Part model, mm, in its own coordinate system. A direction names the side the tool comes from. Round coordinates to 2 decimals unless told otherwise and drop trailing zeros. Write each loop counter-clockwise with the first axis right and the second up, starting at its lowest first coordinate (ties: lowest second). Pieces come first, ordered by that corner, then holes. Notation, with made-up numbers: M -33.75,-4 L -2.75,-4 A30 ccw -2.75,24 Z; hole C 24.25,-1.75 d6. An arc over 180 degrees is marked long. Answer as a JSON object with one key per item and string values. Group by question number.
1. Band-saw the part on A-A, the plane y = 6.75. Write the cut outline in (x, z) (3 decimals).
2. Drill centre lines: line 1 (X direction, y = 1.25, z = -6.75) (3 decimals); line 2 (Z direction, x = 2.75, y = 5); line 3 (Z direction, x = 2.4, y = 4.5). Where is each one in solid material? Low to high. Write a range as from..to.
3. Two-plate mould, pull along Z, no slides. Class faces 1 (the face through (2.724, 1.565, -1.61)), 2 (the face through (0.428, 5.994, -16.053)), 3 (the face through (3, 9.693, -9)), 4 (the face through (2.712, 6.107, -2.265)): +Z half, -Z half, draft (parallel to the pull), parting line (faces both ways), or undercut.
4. Band-saw the part on B-B, the plane z = -7.75. Write the cut outline in (x, y) (3 decimals).
5. Band-saw the part on D-D, the plane z = -2.54. Write the cut outline in (x, y) (3 decimals).
6. Drop a flat-ended pin along its axis: pin 1 (2 mm diameter, centred on y = 4.87, z = -15.47, fed in from +X). Give the stop position or say it passes through.
7. Band-saw the part on C-C, the plane y = 5.75. Write the cut outline in (x, z) (3 decimals), plus the area to 3 significant figures.
8. Which spindle directions (+Z, -Z, +X, -X, +Y, -Y) get a long thin tool onto all of the face, cutting with end or side? Do faces 5 (the face through (0.4, 9.693, -8.9)), 6 (the face through (1.574, 1.915, -16.364)). Say none if no direction does.
Autodesk Inventor part; units mm, degrees
ref_plane "YZ Plane" through (0, 0, 0) normal (1, 0, 0) x (0, 1, 0)
ref_plane "XZ Plane" through (0, 0, 0) normal (0, 1, 0) x (-1, 0, 0)
ref_plane "XY Plane" through (0, 0, 0) normal (0, 0, 1) x (1, 0, 0)
sketch "Sketch1" plane through (0, 0, 0) normal (1, 0, 0) x (0, 1, 0)
  line L0 (0, 0) -> (9.6932, 0)
  line L1 (9.6932, 0) -> (9.6932, -18.0074)
  line L2 (9.6932, -18.0074) -> (0, -18.0074)
  line L3 (0, -18.0074) -> (0, 0)
extrude "Extrusion1" add sketch "Sketch1" along normal blind 3.175
chamfer "Chamfer1" distance 3.175 angle 45 1 edges at (1.5875, 0, 0)
chamfer "Chamfer2" distance 3.175 angle 45 1 edges at (1.5875, 0, -18.0074)
sketch "Sketch2" plane through (0, 9.6932, 0) normal (0, 0, 1) x (1, 0, 0)
  line L0 (0, 0) -> (3.175, 0)
  line L1 (1.5875, 0) -> (0.8676, 0)
  line L2 (0.8676, 0) -> (0.8676, -11.3231)
  line L3 (0.8676, -11.3231) -> (1.5875, -11.3231)
  line L4 (1.5875, -11.3231) -> (1.5875, 0)
  line L5 (1.5875, 0) -> (2.2609, 0)
  line L6 (2.2609, 0) -> (2.2609, -11.3231)
  line L7 (2.2609, -11.3231) -> (1.5875, -11.3231)
  line L8 (1.5875, -11.3231) -> (1.5875, 0)
  point P0 (0, -9.6932)
extrude "Extrusion2" cut sketch "Sketch2" against normal blind 254
ref_plane "Work Plane1" through (3.2004, 0, 0) normal (1, 0, 0) x (0, 0, -1)
sketch "Sketch3" plane through (3.2004, 0, 0) normal (1, 0, 0) x (0, 0, -1)
  circle A0 centre (9.2621, 8.5805) radius 0.766
  point P0 (0, 0)
extrude "Extrusion3" add sketch "Sketch3" against normal blind 3.175
sketch "Sketch4" plane through (3.175, 0, 0) normal (1, 0, 0) x (0, 0, -1)
  circle A0 centre (4.9587, 2.3914) radius 0.8506
  point P0 (0, 0)
extrude "Extrusion4" add sketch "Sketch4" against normal blind 3.175
thicken "Thicken1" operation add thickness 0.0254 both sides no extend neighbours yes toward (-1, 0, 0) faces at (3.2004, 8.8685, -9.0418)
sketch "Sketch5" plane through (3.175, 3.175, -18.0074) normal (1, 0, 0) x (0, 0, -1)
  circle A0 centre (-2.6542, -0.8404) radius 1.0945
  point P0 (-18.0074, -3.175)
extrude "Extrusion5" add sketch "Sketch5" against normal blind 3.175
hole "Hole4" at (3.175, 4.8672, -2.54) direction (-1, 0, 0) diameter 2.54 depth 25.4 tip angle 118
sketch "Sketch6" plane through (3.175, 3.175, -18.0074) normal (1, 0, 0) x (0, 0, -1)
  point P0 (-18.0074, -3.175)
hole "Hole5" at (3.175, 4.8672, -15.4674) direction (-1, 0, 0) diameter 2.54 depth 25.4 tip angle 118
properties part number "gabetrain"
Worked answers:
{
 "1": {"outline": "M 0,-18.007 L 0.868,-18.007 L 0.868,0 L 0,0 Z; M 2.261,-18.007 L 3.175,-18.007 L 3.175,0 L 2.261,0 Z"},
 "2": {"line 1": "x = 0..0.868, 2.261..3.175", "line 2": "z = -18.01..-16.73, -14.2..-3.8, -1.28..0", "line 3": "z = -18.01..-16.68, -14.25..-3.76, -1.32..0"},
 "3": {"face 1": "+Z half", "face 2": "undercut", "face 3": "draft", "face 4": "undercut"},
 "4": {"outline": "M 0,0 L 0.868,0 L 0.868,9.693 L 0,9.693 Z; M 2.261,0 L 3.175,0 L 3.175,9.693 L 2.261,9.693 Z"},
 "5": {"outline": "M 0,0.635 L 0.868,0.635 L 0.868,3.597 L 0,3.597 Z; M 0,6.137 L 0.868,6.137 L 0.868,9.693 L 0,9.693 Z; M 2.261,0.635 L 3.175,0.635 L 3.175,3.597 L 2.261,3.597 Z; M 2.261,6.137 L 3.175,6.137 L 3.175,9.693 L 2.261,9.693 Z"},
 "6": {"pin 1": "passes through"},
 "7": {"outline": "M 0,-18.007 L 0.868,-18.007 L 0.868,-16.38 L 0,-16.38 Z; M 0,-14.554 L 0.868,-14.554 L 0.868,-3.453 L 0,-3.453 Z; M 0,-1.627 L 0.868,-1.627 L 0.868,0 L 0,0 Z; M 2.261,-18.007 L 3.175,-18.007 L 3.175,-16.38 L 2.261,-16.38 Z; M 2.261,-14.554 L 3.175,-14.554 L 3.175,-3.453 L 2.261,-3.453 Z; M 2.261,-1.627 L 3.175,-1.627 L 3.175,0 L 2.261,0 Z", "area": "25.6 mm^2"},
 "8": {"face 5": "+Z, -Z, +X, -X, +Y", "face 6": "none"}
}
